```python
from build123d import *

# Parameters (mm, degrees)
SKIZZE1_R                                   = 22.5
SKIZZE1_R_2                                 = 4.818475195
SKIZZE1_R_3                                 = 2
AUFSATZ_LINEAR_AUSTRAGEN1_DEPTH             = 5
VERRUNDUNG1_R                               = 1
VERRUNDUNG2_R                               = 0.5
FORMSENKUNG_F_R_M4_SENKSCHRAUBE_MIT_2_COUNT = 2
FORMSENKUNG_F_R_M4_SENKSCHRAUBE_MIT_2_PITCH = 23
FORMSENKUNG_F_R_M4_SENKSCHRAUBE_MIT_3_COUNT = 2
FORMSENKUNG_F_R_M4_SENKSCHRAUBE_MIT_3_PITCH = 23
FORMSENKUNG_F_R_M4_SENKSCHRAUBE_MIT_4_COUNT = 2
FORMSENKUNG_F_R_M4_SENKSCHRAUBE_MIT_4_PITCH = 32.526911935


with BuildPart() as part:
    # Skizze1 → Aufsatz-Linear austragen1 (new body)
    with BuildSketch(Plane.XY):
        Circle(SKIZZE1_R)
        Circle(SKIZZE1_R_2, mode=Mode.SUBTRACT)
        with Locations((-11.5, 11.5)):
            Circle(SKIZZE1_R_3, mode=Mode.SUBTRACT)
        with Locations((11.5, 11.5)):
            Circle(SKIZZE1_R_3, mode=Mode.SUBTRACT)
        with Locations((-11.5, -11.5)):
            Circle(SKIZZE1_R_3, mode=Mode.SUBTRACT)
        with Locations((11.5, -11.5)):
            Circle(SKIZZE1_R_3, mode=Mode.SUBTRACT)
    extrude(amount=AUFSATZ_LINEAR_AUSTRAGEN1_DEPTH)

    # Verrundung1
    verrundung1_edges = [part.edges().sort_by_distance(p)[0] for p in [
        (-22.5, 0, 0),
    ]]
    fillet(verrundung1_edges, radius=VERRUNDUNG1_R)

    # Verrundung2
    verrundung2_edges = [part.edges().sort_by_distance(p)[0] for p in [
        (-4.818475195, 0, 0),
    ]]
    fillet(verrundung2_edges, radius=VERRUNDUNG2_R)

    # Skizze2 → Formsenkung für M4 Senkschraube mit Innensechskant1 (revolve, cut)
    with BuildSketch(Plane(origin=(11.5, 11.5, 0), x_dir=(0, 1, 0), z_dir=(1, 0, 0))):
        Polygon((0, 0), (0, 5), (2.275, 5), (2.25, 4.975), (2.25, 2.34), (4.59, 0), align=None)
    formsenkung_f_r_m4_senkschraube_mit_inne = revolve(axis=Axis((11.5, 11.5, -6.35), (0, 0, 1)), mode=Mode.SUBTRACT)

    # Formsenkung f_r M4 Senkschraube mit  2: Formsenkung für M4 Senkschraube mit Innensechskant1 ×2
    with Locations(*[(-i * FORMSENKUNG_F_R_M4_SENKSCHRAUBE_MIT_2_PITCH, 0, 0) for i in range(1, FORMSENKUNG_F_R_M4_SENKSCHRAUBE_MIT_2_COUNT)]):
        add(formsenkung_f_r_m4_senkschraube_mit_inne, mode=Mode.SUBTRACT)

    # Formsenkung f_r M4 Senkschraube mit  3: Formsenkung für M4 Senkschraube mit Innensechskant1 ×2
    with Locations(*[(0, -i * FORMSENKUNG_F_R_M4_SENKSCHRAUBE_MIT_3_PITCH, 0) for i in range(1, FORMSENKUNG_F_R_M4_SENKSCHRAUBE_MIT_3_COUNT)]):
        add(formsenkung_f_r_m4_senkschraube_mit_inne, mode=Mode.SUBTRACT)

    # Formsenkung f_r M4 Senkschraube mit  4: Formsenkung für M4 Senkschraube mit Innensechskant1 ×2
    with Locations(*[Vector(-0.7071067811865476, -0.7071067811865476, 0) * (i * FORMSENKUNG_F_R_M4_SENKSCHRAUBE_MIT_4_PITCH) for i in range(1, FORMSENKUNG_F_R_M4_SENKSCHRAUBE_MIT_4_COUNT)]):
        add(formsenkung_f_r_m4_senkschraube_mit_inne, mode=Mode.SUBTRACT)


solid = part.part
```
Geometry check sheet. Reference: the model listing, model coordinates, mm. Give positions to 0.01 mm unless a question says otherwise; leave off trailing zeros. Order: outer loops, then holes, each group sorted by start corner. A loop starts at its lowest first (then second) coordinate and runs counter-clockwise, first axis right, second up. Notation, with made-up numbers: (54.25, 58.5) - (92.25, 58.5) arc R19 cw to (92.25, 73.5) - close; hole circle Ø7 at (83, -18.5). An arc over 180 degrees is marked (long way). Answer in a Markdown table with one row per item. Add a question column.
Q1. Cross-section at D-D, the plane y = 11.5. Count the separate pieces of the cut face and the enclosed holes in it, then the cut area to 3 significant figures.
Q2. Gauge pin test, flat ends, axial feed: pin 1 (4 mm diameter, centred on x = -11.5, y = 11.5, fed in from -Z); pin 2 (5 mm diameter, centred on x = -11.5, y = -11.5, fed in from -Z); pin 3 (7 mm diameter, centred on x = 11.5, y = -11.5, fed in from -Z); pin 4 (1.5 mm diameter, centred on y = -17, z = 2, fed in from +X). Record the tip position at first contact, or that the pin passes through.
Q3. Mould release check, pull along Y, two halves, no side actions. Record for faces 1 (the conical face through (13.839, 10.981, 2.194)), 2 (the flat face through (0, 5, 5)), 3 (the cylindrical face through (10.382, -19.961, 2.972)): pulls with the +Y half, pulls with the -Y half, needs draft (parallel to the pull), parting line crosses it, or undercut.
Q4. Cross-section at A-A, the plane x = 0. Enter the section's corners in (y, z), then the cut area to 3 significant figures.
Q5. Cross-section at C-C, the plane z = 3.7. Enter the section's corners in (x, y), then the cut area to 3 significant figures.
Q6. Material ranges on probe 1 along Y at (x, z) = (-13, 2.05); probe 2 along X at (y, z) = (11.5, 3.65); probe 3 along Y at (x, z) = (10, 3.8), recorded low to high. Write a range as from..to.
Check values:
| question | item | result |
|---|---|---|
| 1 | separate pieces | 3 |
| 1 | enclosed holes | 0 |
| 1 | area | 137 mm^2 |
| 2 | pin 1 | passes through |
| 2 | pin 2 | stops at z = 2.09 |
| 2 | pin 3 | stops at z = 1.09 |
| 2 | pin 4 | stops at x = 15.56 |
| 3 | face 1 | undercut |
| 3 | face 2 | needs draft |
| 3 | face 3 | parting line crosses it |
| 4 | outline | (-22.5, 1) arc R1 ccw to (-21.5, 0) - (-5.32, 0) arc R0.5 ccw to (-4.82, 0.5) - (-4.82, 5) - (-22.5, 5) - close; (4.82, 0.5) arc R0.5 ccw to (5.32, 0) - (21.5, 0) arc R1 ccw to (22.5, 1) - (22.5, 5) - (4.82, 5) - close |
| 4 | area | 176 mm^2 |
| 5 | outline | circle Ø45 at (0, 0); hole circle Ø4.5 at (-11.5, -11.5); hole circle Ø4.5 at (-11.5, 11.5); hole circle Ø9.64 at (0, 0); hole circle Ø4.5 at (11.5, -11.5); hole circle Ø4.5 at (11.5, 11.5) |
| 5 | area | 1,450 mm^2 |
| 6 | probe 1 | y = -18.36..-13.55, -9.45..9.45, 13.55..18.36 |
| 6 | probe 2 | x = -19.34..-13.75, -9.25..9.25, 13.75..19.34 |
| 6 | probe 3 | y = -20.16..-13.18, -9.82..9.82, 13.18..20.16 |
